Check sheet for the modelled part. Datum: model origin and axes. Units: mm. Face numbers are marked on the shaded views. Round coordinates to 2 decimals unless told otherwise and drop trailing zeros. Order: outer loops, then holes, each group sorted by start corner. A loop starts at its lowest first (then second) coordinate and runs counter-clockwise, first axis right, second up.
Autodesk Inventor part; units mm, degrees
ref_plane "YZ Plane" through (0, 0, 0) normal (1, 0, 0) x (0, 1, 0)
ref_plane "XZ Plane" through (0, 0, 0) normal (0, 1, 0) x (-1, 0, 0)
ref_plane "XY Plane" through (0, 0, 0) normal (0, 0, 1) x (1, 0, 0)
sketch "Sketch1" plane through (0, 0, 0) normal (0, 1, 0) x (-1, 0, 0)
  circle A0 centre (0, 0) radius 3
  circle A1 centre (0, 0) radius 1.7
  dimension "d0" = 6
  dimension "d3" = 3.4
extrude "Extrusion1" add sketch "Sketch1" along normal blind 6.9 contours A0 | A1
extrude "Extrusion2" cut sketch "Sketch1" along normal blind 3.1 contours A1
sketch "Sketch2" plane through (0, 6.9, 0) normal (0, 1, 0) x (1, 0, 0)
  circle A0 centre (0, 0) radius 1.7
extrude "Extrusion3" cut sketch "Sketch2" against normal blind 3.1
sketch "Sketch3" plane through (0, 3.8, 0) normal (0, 1, 0) x (1, 0, 0)
  line L0 (1, 2) -> (-1, 2)
  line L1 (-1, 2) -> (-1, -2)
  line L2 (-1, -2) -> (1, -2)
  line L3 (1, -2) -> (1, 2)
  line L4 (1, 2) -> (-1, -2) construction
  line L5 (-1, 2) -> (1, -2) construction
  circle A0 centre (0, 0) radius 1.7
  point P0 (1, -1.3748)
  point P1 (1, 1.3748)
  point P2 (-1, 1.3748)
  point P3 (-1, -1.3748)
  dimension "d8" = 2
extrude "Extrusion4" cut sketch "Sketch3" against normal blind 0.2 contours L3 A0 L1
sketch "Sketch4" plane through (0, 3.1, 0) normal (0, -1, 0) x (1, 0, 0)
  line L0 (1, -1.3748) -> (1, 1.3748)
  arc A0 (-1, -1.3748) -> (1, -1.3748) centre (0, 0) ccw
  line L1 (-1, 1.3748) -> (-1, -1.3748)
  arc A1 (1, 1.3748) -> (-1, 1.3748) centre (0, 0) ccw
extrude "Extrusion5" cut sketch "Sketch4" against normal blind 0.2
properties part number "Printed Standoff 6.9mm"
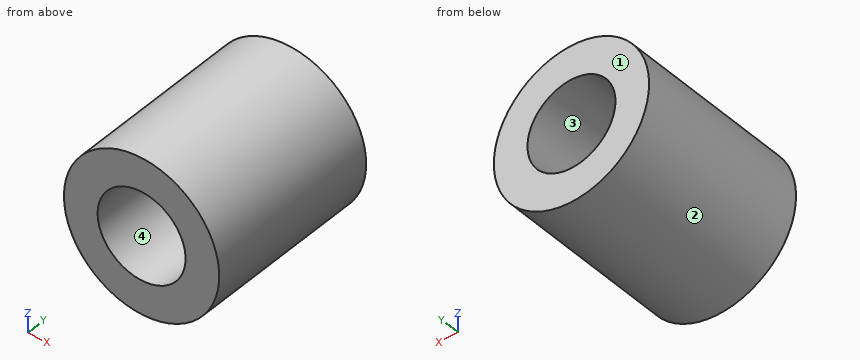
Item 1: Sectioned sample at B-B (y = 4). Record the cut outline in (x, z).
Answer:
outline: circle Ø6 at (0, 0); hole circle Ø3.4 at (0, 0)
Item 2: Scan lines: line 1 along Z through (x, y) = (0.05, 1); line 2 along Y through (x, z) = (1.1, -0.4); line 3 along Z through (x, y) = (-0.8, 2.25). Record each from-to range of solid material in increasing order.
Answer:
line 1: z = -3 to -1.7, 1.7 to 3
line 2: y = 3.1 to 3.8
line 3: z = -2.89 to -1.5, 1.5 to 2.89
Item 3: Go/stop test with flat-tipped pins: P1, Ø2.5, axis at x = 0, z = 0, coming from the +Y side; P2, Ø1.5, axis at x = 2, y = 2.5, coming from the -Z side; P3, Ø1.6, axis at x = 0, z = 0, coming from the +Y side. Record where each tip stops, or that it passes through.
Answer:
P1: stops at y = 3.8
P2: stops at z = -2.73
P3: stops at y = 3.6
Item 4: Sectioned sample at C-C (x = 1.15). Record the cut outline in (y, z), and give its area (3 significant figures).
Answer:
outline: (0, -2.77) - (6.9, -2.77) - (6.9, -1.25) - (3.8, -1.25) - (3.8, 1.25) - (6.9, 1.25) - (6.9, 2.77) - (0, 2.77) - (0, 1.25) - (3.1, 1.25) - (3.1, -1.25) - (0, -1.25) - close
area: 22.7 mm2
Item 5: Release check for a two-part mould opening along Z. For the marked faces 1, 2, 3 and 4 record: released by +Z, released by -Z, zero draft, split by the parting line, or undercut.
Answer:
face 1: zero draft
face 2: split by the parting line
face 3: undercut
face 4: undercut
Item 6: Sectioned sample at A-A (z = 0). Record the cut outline in (x, y), and give its area (3 significant figures).
Answer:
outline: (-3, 0) - (-1.7, 0) - (-1.7, 3.1) - (-1, 3.1) - (-1, 3.3) - (1, 3.3) - (1, 3.1) - (1.7, 3.1) - (1.7, 0) - (3, 0) - (3, 6.9) - (1.7, 6.9) - (1.7, 3.8) - (1, 3.8) - (1, 3.6) - (-1, 3.6) - (-1, 3.8) - (-1.7, 3.8) - (-1.7, 6.9) - (-3, 6.9) - close
area: 19.5 mm2
Item 7: Sectioned sample at D-D (x = -1.1). Record the cut outline in (y, z), and give its area (3 significant figures).
Answer:
outline: (0, -2.79) - (6.9, -2.79) - (6.9, -1.3) - (3.8, -1.3) - (3.8, 1.3) - (6.9, 1.3) - (6.9, 2.79) - (0, 2.79) - (0, 1.3) - (3.1, 1.3) - (3.1, -1.3) - (0, -1.3) - close
area: 22.4 mm2
